Check sheet for the drawn part. Datum: minimum x, y, z corner. Units: mm. Round coordinates to 2 decimals unless told otherwise and drop trailing zeros. Loops run counter-clockwise (first coordinate to the right, second up) from the corner with the lowest first, then second, coordinate; pieces in that order, holes last. Notation, with made-up numbers: (33, -36) -> (45, -36) arc R31 ccw to (45, -5) -> close; hole circle Ø2 at (72.5, 3.25). An arc over 180 degrees is marked (long way). Return JSON: item names as keys, results as strings.
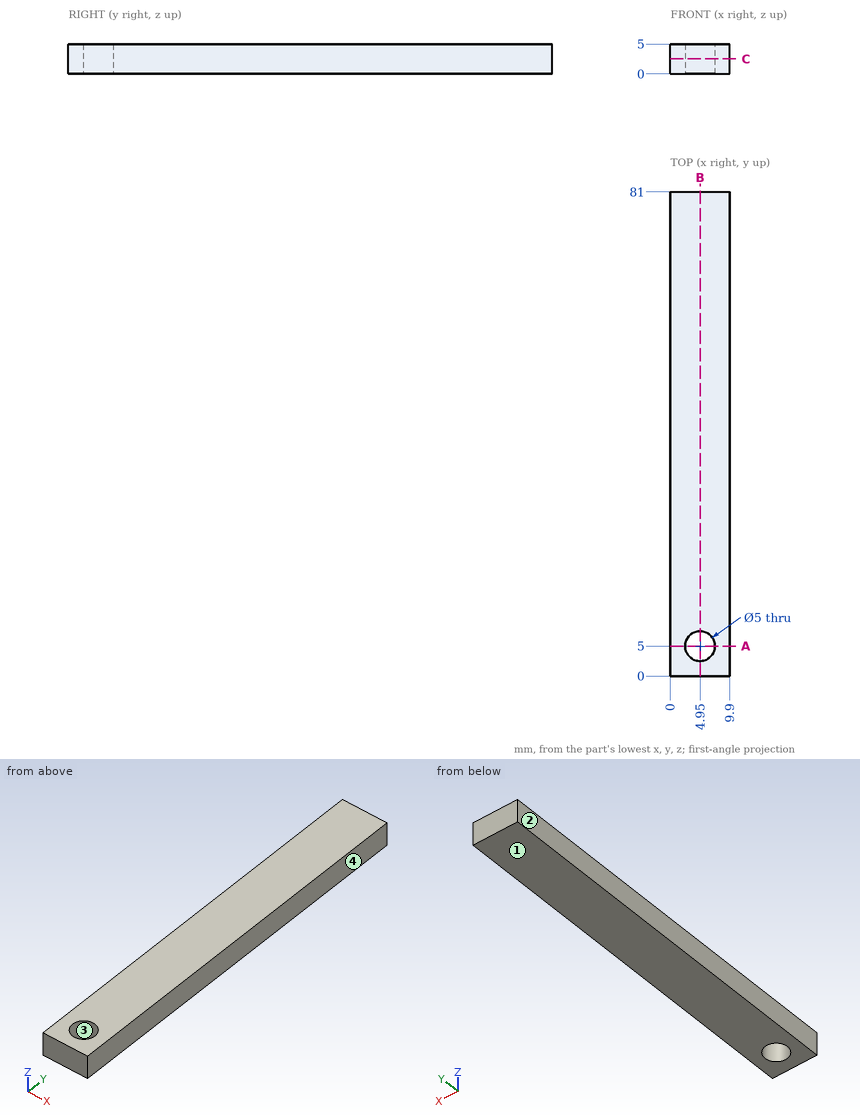
Q1. Material ranges on line 1 (Y direction, x = 4.95, z = 3.25); line 2 (X direction, y = 5, z = 4.05); line 3 (Y direction, x = 3.25, z = 3.1), recorded low to high.
Results list:
{"line 1": "0 to 2.5, 7.5 to 81", "line 2": "0 to 2.45, 7.45 to 9.9", "line 3": "0 to 3.17, 6.83 to 81"}
Q2. Section check B-B (x = 4.95). Record the boundary of the cut face in (y, z), then the cut area to 3 significant figures.
Results list:
{"outline": "(0, 0) -> (2.5, 0) -> (2.5, 5) -> (0, 5) -> close; (7.5, 0) -> (81, 0) -> (81, 5) -> (7.5, 5) -> close", "area": "380 mm^2"}
Q3. Draft check along X on the marked faces 1, 2, 3 and 4. Enter one of: released by +X, released by -X, zero draft, split by the parting line, or undercut.
Results list:
{"face 1": "zero draft", "face 2": "released by -X", "face 3": "undercut", "face 4": "released by +X"}
Q4. Section check A-A (y = 5). Record the boundary of the cut face in (x, z).
Results list:
{"outline": "(0, 0) -> (2.45, 0) -> (2.45, 5) -> (0, 5) -> close; (7.45, 0) -> (9.9, 0) -> (9.9, 5) -> (7.45, 5) -> close"}
Q5. Section check C-C (z = 2.5). Record the boundary of the cut face in (x, y), then the cut area to 3 significant figures.
Results list:
{"outline": "(0, 0) -> (9.9, 0) -> (9.9, 81) -> (0, 81) -> close; hole circle Ø5 at (4.95, 5)", "area": "782 mm^2"}
